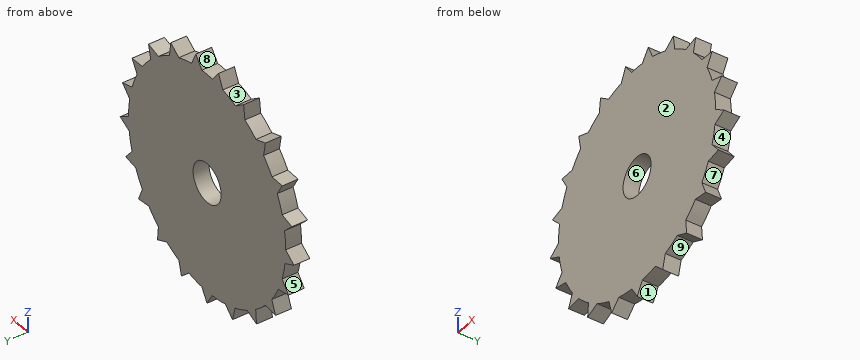
```python
from build123d import *

# Parameters (mm, degrees)
F0_R     = 7.9375
F1_DEPTH = 6.35


with BuildPart() as f1:
    # F0 (on Front) → F1 (new body)
    with BuildSketch(Plane.XZ):
        with BuildLine():
            ThreePointArc((44.0640721068, -5.844659902), (44.3534130882, -2.9286938091), (44.45, 0))
            ThreePointArc((44.45, 0), (44.2916429403, 3.7487151993), (43.8177000834, 7.4707201392))
            ThreePointArc((43.8177000834, 7.4707201392), (43.2302609799, 10.3415199856), (42.4549488772, 13.1673769534))
            ThreePointArc((42.4549488772, 13.1673769534), (41.1932213858, 16.7009284729), (39.6379848993, 20.1154829204))
            ThreePointArc((39.6379848993, 20.1154829204), (38.2264978161, 22.6834160724), (36.6488834271, 25.1527700969))
            ThreePointArc((36.6488834271, 25.1527700969), (34.3970458346, 28.1539648691), (31.900123201, 30.9545576574))
            ThreePointArc((31.900123201, 30.9545576574), (29.7912918003, 32.9891108226), (27.552991384, 34.8802976735))
            ThreePointArc((27.552991384, 34.8802976735), (24.5131823233, 37.0797302092), (21.2987124989, 39.0149631025))
            ThreePointArc((21.2987124989, 39.0149631025), (20.0011436472, 39.6958027102), (18.6818383084, 40.3335024194))
            Line((18.6818383084, 40.3335024194), (15.9837753185, 41.476757667))
            ThreePointArc((15.9837753185, 41.476757667), (12.4288665323, 42.6769935296), (8.7853998717, 43.5731482578))
            Line((8.7853998717, 43.5731482578), (5.8953894288, 44.0573136208))
            ThreePointArc((5.8953894288, 44.0573136208), (4.4399865206, 44.227695166), (2.9797584028, 44.3500117233))
            ThreePointArc((2.9797584028, 44.3500117233), (-0.0511777408, 44.4499705381), (-3.0818756726, 44.3430326245))
            ThreePointArc((-3.0818756726, 44.3430326245), (-5.99682497, 44.0436214483), (-8.8857128589, 43.5528025159))
            ThreePointArc((-8.8857128589, 43.5528025159), (-12.5271062762, 42.6482603203), (-16.0792418436, 41.4398417195))
            ThreePointArc((-16.0792418436, 41.4398417195), (-18.7746650962, 40.2903766491), (-21.3884961364, 38.9658149282))
            ThreePointArc((-21.3884961364, 38.9658149282), (-24.5985011604, 37.0231851772), (-27.6332375088, 34.8167586772))
            ThreePointArc((-27.6332375088, 34.8167586772), (-29.8671771379, 32.9204226858), (-31.9713179637, 30.8810188896))
            ThreePointArc((-31.9713179637, 30.8810188896), (-34.4617850273, 28.0746838403), (-36.7067057715, 25.0683116983))
            ThreePointArc((-36.7067057715, 25.0683116983), (-38.2786297743, 22.5953314338), (-39.6841999125, 20.0241548461))
            ThreePointArc((-39.6841999125, 20.0241548461), (-41.2315695506, 16.6060281944), (-42.4851569561, 13.0695806519))
            ThreePointArc((-42.4851569561, 13.0695806519), (-43.253959877, 10.2419458581), (-43.8347868066, 7.3698009215))
            ThreePointArc((-43.8347868066, 7.3698009215), (-44.3001577128, 3.6467144971), (-44.4498821525, -0.1023554137))
            ThreePointArc((-44.4498821525, -0.1023554137), (-44.3465515673, -3.0308190466), (-44.0504967316, -5.9461111405))
            ThreePointArc((-44.0504967316, -5.9461111405), (-43.3920943841, -9.6399504647), (-42.424515682, -13.2651034351))
            ThreePointArc((-42.424515682, -13.2651034351), (-41.4583271722, -16.0315192069), (-40.3119662534, -18.7282641156))
            ThreePointArc((-40.3119662534, -18.7282641156), (-38.5888928498, -22.0612748641), (-36.5908667529, -25.2370951235))
            ThreePointArc((-36.5908667529, -25.2370951235), (-34.8485512733, -27.5931327354), (-32.954788597, -29.8292542402))
            ThreePointArc((-32.954788597, -29.8292542402), (-30.3217176818, -32.5022451044), (-27.4725991601, -34.943651718))
            ThreePointArc((-27.4725991601, -34.943651718), (-25.1105575411, -36.6778189097), (-22.6393887587, -38.2525891494))
            ThreePointArc((-22.6393887587, -38.2525891494), (-19.3326807859, -40.025616218), (-15.8882240398, -41.5134536851))
            ThreePointArc((-15.8882240398, -41.5134536851), (-13.1184874977, -42.4700810662), (-10.2917397433, -43.2421390897))
            ThreePointArc((-10.2917397433, -43.2421390897), (-6.6082249244, -43.9560446736), (-2.877625333, -44.3567556573))
            ThreePointArc((-2.877625333, -44.3567556573), (0.0511777408, -44.4499705381), (2.9797584028, -44.3500117233))
            ThreePointArc((2.9797584028, -44.3500117233), (6.7094253828, -43.9407113169), (10.391286519, -43.2183255631))
            ThreePointArc((10.391286519, -43.2183255631), (13.2162489541, -42.4397604091), (15.9837753185, -41.476757667))
            ThreePointArc((15.9837753185, -41.476757667), (19.4247968758, -39.9809925631), (22.7274133165, -38.2003558091))
            ThreePointArc((22.7274133165, -38.2003558091), (25.1949493097, -36.619899362), (27.552991384, -34.8802976735))
            ThreePointArc((27.552991384, -34.8802976735), (30.3964805031, -32.4323368419), (33.0233893173, -29.7532898685))
            ThreePointArc((33.0233893173, -29.7532898685), (34.9119978358, -27.5128135078), (36.6488834271, -25.1527700969))
            ThreePointArc((36.6488834271, -25.1527700969), (38.6395912369, -21.9723573847), (40.3549851186, -18.6353877362))
            ThreePointArc((40.3549851186, -18.6353877362), (40.9473091431, -17.2950968178), (41.4951331794, -15.9360102417))
            Line((41.4951331794, -15.9360102417), (42.4549488772, -13.1673769534))
            ThreePointArc((42.4549488772, -13.1673769534), (43.4141773417, -9.5400055419), (44.0640721068, -5.844659902))
        make_face()
        Circle(F0_R, mode=Mode.SUBTRACT)
        with BuildLine():
            Line((49.1725476546, -3.0876265469), (44.45, 0))
            ThreePointArc((44.45, 0), (44.3534130882, -2.9286938091), (44.0640721068, -5.844659902))
            Line((44.0640721068, -5.844659902), (49.1725476546, -3.0876265469))
        make_face()
        with BuildLine():
            ThreePointArc((42.4549488772, 13.1673769534), (43.2302609799, 10.3415199856), (43.8177000834, 7.4707201392))
            Line((43.8177000834, 7.4707201392), (47.8801786158, 11.6172878184))
            Line((47.8801786158, 11.6172878184), (42.4549488772, 13.1673769534))
        make_face()
        with BuildLine():
            Line((46.0508898584, -17.5153767813), (42.4549488772, -13.1673769534))
            ThreePointArc((42.4549488772, -13.1673769534), (41.997861873, -14.5596050118), (41.4951331794, -15.9360102417))
            ThreePointArc((41.4951331794, -15.9360102417), (40.9473091431, -17.2950968178), (40.3549851186, -18.6353877362))
            Line((40.3549851186, -18.6353877362), (46.0508898584, -17.5153767813))
        make_face()
        with BuildLine():
            ThreePointArc((41.4951331794, -15.9360102417), (41.997861873, -14.5596050118), (42.4549488772, -13.1673769534))
            Line((42.4549488772, -13.1673769534), (41.4951331794, -15.9360102417))
        make_face()
        with BuildLine():
            ThreePointArc((36.6488834271, 25.1527700969), (38.2264978161, 22.6834160724), (39.6379848993, 20.1154829204))
            Line((39.6379848993, 20.1154829204), (42.4520045518, 25.0060030808))
            Line((42.4520045518, 25.0060030808), (36.6488834271, 25.1527700969))
        make_face()
        with BuildLine():
            ThreePointArc((27.552991384, 34.8802976735), (29.7912918003, 32.9891108226), (31.900123201, 30.9545576574))
            Line((31.900123201, 30.9545576574), (33.1391274312, 36.4591705012))
            Line((33.1391274312, 36.4591705012), (27.552991384, 34.8802976735))
        make_face()
        with BuildLine():
            Line((38.7954242099, -30.3708403064), (36.6488834271, -25.1527700969))
            ThreePointArc((36.6488834271, -25.1527700969), (34.9119978358, -27.5128135078), (33.0233893173, -29.7532898685))
            Line((33.0233893173, -29.7532898685), (38.7954242099, -30.3708403064))
        make_face()
        with BuildLine():
            ThreePointArc((18.6818383084, 40.3335024194), (20.0011436472, 39.6958027102), (21.2987124989, 39.0149631025))
            Line((21.2987124989, 39.0149631025), (20.5630526794, 44.7731364218))
            Line((20.5630526794, 44.7731364218), (15.9837753185, 41.476757667))
            ThreePointArc((15.9837753185, 41.476757667), (17.3422302537, 40.9273692024), (18.6818383084, 40.3335024194))
        make_face()
        with BuildLine():
            Line((28.0574454172, -40.500032558), (27.552991384, -34.8802976735))
            ThreePointArc((27.552991384, -34.8802976735), (25.1949493097, -36.619899362), (22.7274133165, -38.2003558091))
            Line((22.7274133165, -38.2003558091), (28.0574454172, -40.500032558))
        make_face()
        with BuildLine():
            Line((15.9837753185, 41.476757667), (18.6818383084, 40.3335024194))
            ThreePointArc((18.6818383084, 40.3335024194), (17.3422302537, 40.9273692024), (15.9837753185, 41.476757667))
        make_face()
        with BuildLine():
            Line((14.4973696484, -47.0882061011), (15.9837753185, -41.476757667))
            ThreePointArc((15.9837753185, -41.476757667), (13.2162489541, -42.4397604091), (10.391286519, -43.2183255631))
            Line((10.391286519, -43.2183255631), (14.4973696484, -47.0882061011))
        make_face()
        with BuildLine():
            Line((5.8953894288, 44.0573136208), (8.7853998717, 43.5731482578))
            ThreePointArc((8.7853998717, 43.5731482578), (7.3443854505, 43.839052252), (5.8953894288, 44.0573136208))
        make_face()
        with BuildLine():
            ThreePointArc((5.8953894288, 44.0573136208), (7.3443854505, 43.839052252), (8.7853998717, 43.5731482578))
            Line((8.7853998717, 43.5731482578), (6.3770210487, 48.8549535164))
            Line((6.3770210487, 48.8549535164), (2.9797584028, 44.3500117233))
            ThreePointArc((2.9797584028, 44.3500117233), (4.4399865206, 44.227695166), (5.8953894288, 44.0573136208))
        make_face()
        with BuildLine():
            Line((0.0511777408, -49.2717251549), (2.9797584028, -44.3500117233))
            ThreePointArc((2.9797584028, -44.3500117233), (0.0511777408, -44.4499705381), (-2.877625333, -44.3567556573))
            Line((-2.877625333, -44.3567556573), (0.0511777408, -49.2717251549))
        make_face()
        with BuildLine():
            ThreePointArc((-8.8857128589, 43.5528025159), (-5.99682497, 44.0436214483), (-3.0818756726, 44.3430326245))
            Line((-3.0818756726, 44.3430326245), (-6.4895028814, 48.8401395667))
            Line((-6.4895028814, 48.8401395667), (-8.8857128589, 43.5528025159))
        make_face()
        with BuildLine():
            Line((-14.3889007778, -47.1214644822), (-10.2917397433, -43.2421390897))
            ThreePointArc((-10.2917397433, -43.2421390897), (-13.1184874977, -42.4700810662), (-15.8882240398, -41.5134536851))
            Line((-15.8882240398, -41.5134536851), (-14.3889007778, -47.1214644822))
        make_face()
        with BuildLine():
            ThreePointArc((-21.3884961364, 38.9658149282), (-18.7746650962, 40.2903766491), (-16.0792418436, 41.4398417195))
            Line((-16.0792418436, 41.4398417195), (-20.6660976647, 44.7256669917))
            Line((-20.6660976647, 44.7256669917), (-21.3884961364, 38.9658149282))
        make_face()
        with BuildLine():
            Line((-27.964111242, -40.564533314), (-22.6393887587, -38.2525891494))
            ThreePointArc((-22.6393887587, -38.2525891494), (-25.1105575411, -36.6778189097), (-27.4725991601, -34.943651718))
            Line((-27.4725991601, -34.943651718), (-27.964111242, -40.564533314))
        make_face()
        with BuildLine():
            ThreePointArc((-31.9713179637, 30.8810188896), (-29.8671771379, 32.9204226858), (-27.6332375088, 34.8167586772))
            Line((-27.6332375088, 34.8167586772), (-32.9875778767, 36.596346626))
            Line((-32.9875778767, 36.596346626), (-31.9713179637, 30.8810188896))
        make_face()
        with BuildLine():
            Line((-38.7253861476, -30.4600943574), (-32.954788597, -29.8292542402))
            ThreePointArc((-32.954788597, -29.8292542402), (-34.8485512733, -27.5931327354), (-36.5908667529, -25.2370951235))
            Line((-36.5908667529, -25.2370951235), (-38.7253861476, -30.4600943574))
        make_face()
        with BuildLine():
            ThreePointArc((-39.6841999125, 20.0241548461), (-38.2786297743, 22.5953314338), (-36.7067057715, 25.0683116983))
            Line((-36.7067057715, 25.0683116983), (-42.509473549, 24.9081821723))
            Line((-42.509473549, 24.9081821723), (-39.6841999125, 20.0241548461))
        make_face()
        with BuildLine():
            Line((-46.0104349513, -17.621372141), (-40.3119662534, -18.7282641156))
            ThreePointArc((-40.3119662534, -18.7282641156), (-41.4583271722, -16.0315192069), (-42.424515682, -13.2651034351))
            Line((-42.424515682, -13.2651034351), (-46.0104349513, -17.621372141))
        make_face()
        with BuildLine():
            ThreePointArc((-43.8347868066, 7.3698009215), (-43.253959877, 10.2419458581), (-42.4851569561, 13.0695806519))
            Line((-42.4851569561, 13.0695806519), (-47.906802907, 11.5070029014))
            Line((-47.906802907, 11.5070029014), (-43.8347868066, 7.3698009215))
        make_face()
        with BuildLine():
            Line((-49.1436337538, -3.5179741351), (-44.0504967316, -5.9461111405))
            ThreePointArc((-44.0504967316, -5.9461111405), (-44.3465515673, -3.0308190466), (-44.4498821525, -0.1023554137))
            Line((-44.4498821525, -0.1023554137), (-49.1436337538, -3.5179741351))
        make_face()
    extrude(amount=F1_DEPTH)


solid = f1.part
```
The model under review builds one solid part; all positions refer to its coordinate system, in mm. Face numbers are marked on the shaded views. A direction names the side the tool comes from. Round coordinates to 2 decimals unless told otherwise and drop trailing zeros. Write each loop counter-clockwise with the first axis right and the second up, starting at its lowest first coordinate (ties: lowest second). Pieces come first, ordered by that corner, then holes. Notation, with made-up numbers: M 11,66 L 64,66 A26 cw 64,84 Z; hole C 51,7 d4. An arc over 180 degrees is marked long. Use CSV: the item, a comma, the result in double quotes. Start each with the question number.
(1) The part is to be moulded in two halves that separate along X. For the marked faces 1, 2, 3 and 4, say which applies: +X half, -X half, draft (parallel to the pull), parting line (faces both ways), or undercut.
(2) We need section A-A, the plane x = 25. State the section outline as (y, z) points.
(3) Clearance check with flat-ended pins moving along their axes: P1, Ø1.5, axis at y = -4, z = -21.5, coming from the -X side; P2, Ø12.5, axis at x = 0, z = 0, coming from the +Y side. State where each tip first meets the part, or that it passes through.
(4) Tool access review of the marked faces 5, 6, 7, 8 and 9: name each direction out of +Z, -Z, +X, -X, +Y, -Y from which nothing blocks a thin tool from reaching the whole face with its end or side.
(5) For line 1 along Z through (x, y) = (0, -2.75); line 2 along Z through (x, y) = (4.5, -3.75); line 3 along X through (y, z) = (-3.25, -2.5), list the stretches that pass through material, from the lowest coordinate up.
Findings:
1,face 1,"undercut"
1,face 2,"draft"
1,face 3,"undercut"
1,face 4,"+X half"
2,outline,"M -6.35,-39.18 L 0,-39.18 L 0,36.75 L -6.35,36.75 Z"
3,P1,"x = -39.31"
3,P2,"through"
4,face 5,"-X, +Y, -Y"
4,face 6,"+Y, -Y"
4,face 7,"+X, +Y, -Y"
4,face 8,"+Z, +Y, -Y"
4,face 9,"-Z, +Y, -Y"
5,line 1,"-49.19 to -7.94, 7.94 to 44.45"
5,line 2,"-44.22 to -6.54, 6.54 to 46.37"
5,line 3,"-47.74 to -7.53, 7.53 to 48.27"
